Verification items for the finished model (mm, model axes). A direction names the side the tool comes from. Coordinates: 2 decimals unless noted, no trailing zeros. Loops run counter-clockwise (first coordinate to the right, second up) from the corner with the lowest first, then second, coordinate; pieces in that order, holes last. Notation, with made-up numbers: (-37.5, -1) - (-26.5, -1) arc R17 ccw to (-26.5, 24) - close; hole circle Ø8 at (50.25, -22.5). An arc over 180 degrees is marked (long way). One line per item, written item: value. Start each with the question number.
(1) Section check B-B (x = 0). Record the boundary of the cut face in (y, z).
(2) Thickness scan on probe 1 along Z at (x, y) = (0, 2.5); probe 2 along X at (y, z) = (97.5, -12.5); probe 3 along Y at (x, z) = (20.5, 13). Record the ranges inside material, lowest first. Write a range as [from, to].
(3) Section check A-A (y = 32). Record the boundary of the cut face in (x, z), plus the area to 3 significant figures.
(4) Gauge pin test, flat ends, axial feed: P1, Ø16, axis at y = 117.5, z = 2, coming from the +X side; P2, Ø12, axis at y = 116.5, z = 0, coming from the +X side; P3, Ø1, axis at x = 20.5, z = -7.5, coming from the +Y side; P4, Ø2, axis at x = 18, z = 0, coming from the -Y side. Record the tip position at first contact, or that the pin passes through.
(5) Section check C-C (z = 3). Count the separate pieces of the cut face and the enclosed holes in it, plus the area to 3 significant figures.
(6) Draft check along X on faces 6 (the face through (-24, 39, -9)), 7 (the face through (16, 129, -9)), 8 (the face through (16.5, 119, 7)). Enter one of: +X half, -X half, draft (parallel to the pull), parting line (faces both ways), or undercut.
(7) Set-up check for faces 1 (the face through (-15, 4, -15)), 2 (the face through (-15.23, 110.79, -3.23)), 3 (the face through (-14, 101, -1)), 4 (the face through (17.24, 107.085, 1.302)), 5 (the face through (-17.24, 126.915, 1.302)): record each of +Z, -Z, +X, -X, +Y, -Y from which the full face is reachable in a straight line by a thin tool's end or side.
(8) Section check D-D (z = -29). Record the boundary of the cut face in (x, y), plus the area to 3 significant figures.
Autodesk Inventor part; units mm, degrees
ref_plane "YZ Plane" through (0, 0, 0) normal (1, 0, 0) x (0, 1, 0)
ref_plane "XZ Plane" through (0, 0, 0) normal (0, 1, 0) x (-1, 0, 0)
ref_plane "XY Plane" through (0, 0, 0) normal (0, 0, 1) x (1, 0, 0)
sketch "Sketch1" plane through (0, 0, 0) normal (0, 0, 1) x (1, 0, 0)
  line L0 (-18, 132) -> (-18, 80)
  line L1 (-20, 78) -> (-22, 78)
  line L2 (-28, 72) -> (-28, 6)
  line L3 (-22, 0) -> (22, 0)
  line L4 (28, 6) -> (28, 72)
  line L5 (22, 78) -> (20, 78)
  line L6 (18, 80) -> (18, 132)
  arc A0 (-28, 6) -> (-22, 0) centre (-22, 6) ccw
  arc A1 (-22, 78) -> (-28, 72) centre (-22, 72) ccw
  arc A2 (28, 72) -> (22, 78) centre (22, 72) ccw
  arc A3 (22, 0) -> (28, 6) centre (22, 6) ccw
  arc A4 (-20, 78) -> (-18, 80) centre (-20, 80) ccw
  arc A5 (18, 80) -> (20, 78) centre (20, 80) ccw
  line L7 (-14, 132) -> (-14, 80)
  arc A6 (-20, 74) -> (-14, 80) centre (-20, 80) ccw
  line L8 (-20, 74) -> (-22, 74)
  arc A7 (-22, 74) -> (-24, 72) centre (-22, 72) ccw
  line L9 (-24, 72) -> (-24, 6)
  arc A8 (-24, 6) -> (-22, 4) centre (-22, 6) ccw
  line L10 (-22, 4) -> (22, 4)
  arc A9 (22, 4) -> (24, 6) centre (22, 6) ccw
  line L11 (24, 6) -> (24, 72)
  arc A10 (24, 72) -> (22, 74) centre (22, 72) ccw
  line L12 (22, 74) -> (20, 74)
  arc A11 (14, 80) -> (20, 74) centre (20, 80) ccw
  line L13 (14, 80) -> (14, 132)
  line L14 (14, 132) -> (18, 132)
  line L15 (-14, 132) -> (-18, 132)
  point P0 (0, 0)
  point P1 (0, 0)
  dimension "d0" = 132
  dimension "d1" = 6
  dimension "d2" = 2
  dimension "d3" = 56
  dimension "d4" = 36
  dimension "d5" = 4
  dimension "d6" = 78
extrude "Extrusion1" add sketch "Sketch1" along normal blind 15 and the other way blind 33
fillet "Fillet1" radius 15 2 edges at (-16, 132, 15) (16, 132, 15)
sketch "Sketch3" plane through (0, 0, 0) normal (1, 0, 0) x (0, 1, 0)
  arc A0 (132, 0) -> (117, 15) centre (117, 0) ccw
  line L0 (72, -33) -> (6, -33)
  arc A1 (120.8823, -14.4889) -> (132, 0) centre (117, 0) ccw
  line L1 (120.8823, -14.4889) -> (51.7979, -33)
  line L2 (6, 15) -> (72, 15)
  line L3 (51.7979, -33) -> (132, -33)
  line L4 (132, -33) -> (132, 0)
  point P0 (0, 0)
  dimension "d12" = 15
extrude "Extrusion2" cut sketch "Sketch3" along normal through all both and the other way through all
sketch "Sketch4" plane through (18, 80, 15) normal (1, 0, 0) x (0, 0, -1)
  arc A0 (29.4889, 40.8823) -> (0, 37) centre (15, 37) ccw
  point P0 (15, -80)
hole "Hole1" at (18, 117, 0) direction (-1, 0, 0) diameter 14 depth 4 counterbore diameter 20 counterbore depth 1.5
mirror "Mirror1" about plane through (0, 0, 0) normal (1, 0, 0) of "Hole1"
sketch "Sketch5" plane through (-22, 4, 15) normal (0, 1, 0) x (1, 0, 0)
  line L0 (44, 48) -> (0, 0)
  point P0 (22, 15)
  point P1 (22, 24)
hole "Hole2" at (0, 4, -9) direction (0, -1, 0) diameter 30 end through all
properties part number "Part021. High fork" material "Steel, Carbon"
Responses:
1. outline: (0, -33) - (4, -33) - (4, -24) - (0, -24) - close; (0, 6) - (4, 6) - (4, 15) - (0, 15) - close
2. probe 1: z = [-33, -24], [6, 15]
2. probe 2: x = [-18, -14], [14, 18]
2. probe 3: y = [0, 4], [74, 78]
3. outline: (-28, -33) - (-24, -33) - (-24, 15) - (-28, 15) - close; (24, -33) - (28, -33) - (28, 15) - (24, 15) - close
3. area: 384 mm²
4. P1: stops at x = 18
4. P2: passes through
4. P3: stops at y = 78
4. P4: stops at y = 0
5. separate pieces: 4
5. enclosed holes: 0
5. area: 1,090 mm²
6. face 6: undercut
6. face 7: draft
6. face 8: +X half
7. face 1: +Z, -Z
7. face 2: +X, -X
7. face 3: +Z, -Z, +Y
7. face 4: +X
7. face 5: -X
8. outline: (-28, 6) arc R6 ccw to (-22, 0) - (22, 0) arc R6 ccw to (28, 6) - (28, 66.73) - (24, 66.73) - (24, 6) arc R2 cw to (22, 4) - (-22, 4) arc R2 cw to (-24, 6) - (-24, 66.73) - (-28, 66.73) - close
8. area: 712 mm²
